Here's how the part is built. I have some questions about the finished solid (model axes, mm). Coordinates: 2 decimals unless noted, no trailing zeros. Write each loop counter-clockwise with the first axis right and the second up, starting at its lowest first coordinate (ties: lowest second). Pieces come first, ordered by that corner, then holes.
Item 1: If I drill on line 1 (Z direction, x = -0.25, y = 17); line 2 (Z direction, x = -3.5, y = 17.5), over which ranges is the centre line in solid material (lowest first)?
Item 2: I'm going to push flat-ended pins straight in: pin 1 Ø2 at (x, y) = (-1.5, 9) entering from -Z; pin 2 Ø1.5 at (y, z) = (14, 3) entering from +X; pin 3 Ø4 at (x, y) = (-3, 28.5) entering from +Z. Where does each tip first touch, or does it pass through?
Item 3: If we section it at A-A (y = 6.5): Please give me the cut outline in (x, z).
from build123d import *

# Parameters (mm, degrees)
ESQUISSE1_R             = 4
BOSS_EXTRU_1_DEPTH      = 72
CHANFREIN1_SIZE         = 1
CHANFREIN1_SIZE2        = 0.839099631
CHANFREIN1_PART_2_SIZE  = 1
CHANFREIN1_PART_2_SIZE2 = 0.839099631


with BuildPart() as part:
    # Esquisse1 → Boss.-Extru.1 (new body)
    with BuildSketch(Plane(origin=(0, 0, 0), x_dir=(1, 0, 0), z_dir=(0, 1, 0))):
        Circle(ESQUISSE1_R)
    extrude(amount=BOSS_EXTRU_1_DEPTH)

    # Chanfrein1
    chanfrein1_edges = [part.edges().sort_by_distance(p)[0] for p in [
        (-4, 0, 0),
    ]]
    chanfrein1_side = [part.faces().sort_by_distance(p)[0] for p in [
        (0, 0, 0),
    ]]
    chamfer(chanfrein1_edges, length=CHANFREIN1_SIZE, length2=CHANFREIN1_SIZE2, reference=chanfrein1_side[0])

    # Chanfrein1 part 2
    chanfrein1_part_2_edges = [part.edges().sort_by_distance(p)[0] for p in [
        (-4, 72, 0),
    ]]
    chanfrein1_part_2_side = [part.faces().sort_by_distance(p)[0] for p in [
        (-4, 36, 0),
    ]]
    chamfer(chanfrein1_part_2_edges, length=CHANFREIN1_PART_2_SIZE, length2=CHANFREIN1_PART_2_SIZE2, reference=chanfrein1_part_2_side[0])


solid = part.part
Answer list:
1. line 1: z = -3.99 to 3.99
1. line 2: z = -1.94 to 1.94
2. pin 1: stops at z = -3.97
2. pin 2: stops at x = 3.31
2. pin 3: stops at z = 3.87
3. outline: circle Ø8 at (0, 0)
